Geometry check sheet. Reference: the model listing, model coordinates, mm. Coordinates: 2 decimals unless noted, no trailing zeros. Write each loop counter-clockwise with the first axis right and the second up, starting at its lowest first coordinate (ties: lowest second). Pieces come first, ordered by that corner, then holes. Notation, with made-up numbers: (-25.5, -27.5) -> (-15.5, -27.5) arc R22 cw to (-15.5, -13.5) -> close; hole circle Ø11 at (70, 55). An arc over 180 degrees is marked (long way). One line per question, with ' | ' between items.
from build123d import *

# Parameters (mm, degrees)
SKETCH1_W           = 145
SKETCH1_H           = 155
BOSS_EXTRUDE1_DEPTH = 3
SKETCH3_W           = 4.5
SKETCH3_H           = 4
CUT_EXTRUDE1_DEPTH  = 3
SKETCH4_R           = 2.05
CUT_EXTRUDE2_DEPTH  = 3
SKETCH5_R           = 2.05
CUT_EXTRUDE3_DEPTH  = 10


with BuildPart() as part:
    # Sketch1 → Boss-Extrude1 (new body)
    with BuildSketch(Plane(origin=(0, 0, 0), x_dir=(1, 0, 0), z_dir=(0, 1, 0))):
        Rectangle(SKETCH1_W, SKETCH1_H)
    extrude(amount=BOSS_EXTRUDE1_DEPTH)

    # Sketch3 → Cut-Extrude1 (cut)
    with BuildSketch(Plane(origin=(0, 3, 0), x_dir=(1, 0, 0), z_dir=(0, 1, 0))):
        Polygon((-61.5, -37), (-72.5, -37), (-72.5, -77.5), (-61.5, -77.5), (-61.5, -73.5), align=None)
        with Locations((-59.25, -75.5)):
            Rectangle(SKETCH3_W, SKETCH3_H)
    extrude(amount=-CUT_EXTRUDE1_DEPTH, mode=Mode.SUBTRACT)

    # Sketch4 → Cut-Extrude2 (cut)
    with BuildSketch(Plane(origin=(0, 3, 0), x_dir=(1, 0, 0), z_dir=(0, 1, 0))):
        with Locations(Location((-17.5, -67.5, 0), (0, 0, 270))):
            Circle(SKETCH4_R)
        with Locations(Location((62.5, -67.5, 0), (0, 0, 270))):
            Circle(SKETCH4_R)
        with Locations(Location((-62.5, -22.85, 0), (0, 0, 270))):
            Circle(SKETCH4_R)
        with Locations(Location((-62.5, 57.15, 0), (0, 0, 270))):
            Circle(SKETCH4_R)
        with Locations(Location((62.5, -47.5, 0), (0, 0, 270))):
            Circle(SKETCH4_R)
        with Locations(Location((-17.5, -47.5, 0), (0, 0, 270))):
            Circle(SKETCH4_R)
    extrude(amount=-CUT_EXTRUDE2_DEPTH, mode=Mode.SUBTRACT)

    # Sketch5 → Cut-Extrude3 (cut)
    with BuildSketch(Plane(origin=(0, 3, 0), x_dir=(1, 0, 0), z_dir=(0, 1, 0))):
        with Locations(Location((52.538287268, 25.128851924, 0), (0, 0, 270))):
            Circle(SKETCH5_R)
        with Locations(Location((-14.95509898, 16.575946892, 0), (0, 0, 270))):
            Circle(SKETCH5_R)
    extrude(amount=-CUT_EXTRUDE3_DEPTH, mode=Mode.SUBTRACT)


solid = part.part
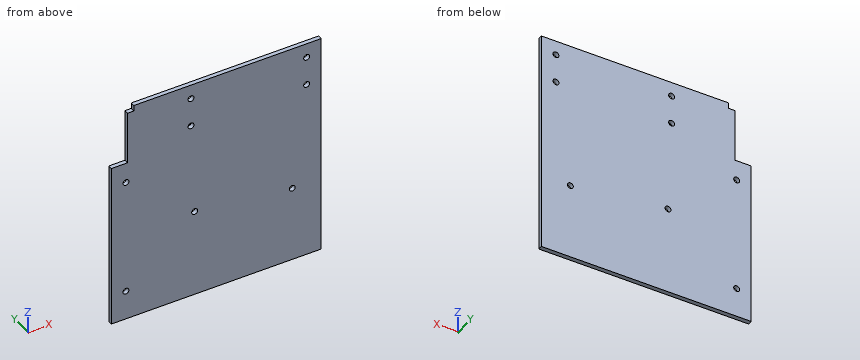
1. Cross-section at B-B on z = 47.5. Record the boundary of the cut face in (x, y).
Worked answers:
outline: (-61.5, 0) -> (-19.55, 0) -> (-19.55, 3) -> (-61.5, 3) -> close; (-15.45, 0) -> (60.45, 0) -> (60.45, 3) -> (-15.45, 3) -> close; (64.55, 0) -> (72.5, 0) -> (72.5, 3) -> (64.55, 3) -> close
2. Cross-section at A-A on x = 62.5. Record the boundary of the cut face in (y, z).
Worked answers:
outline: (0, -77.5) -> (3, -77.5) -> (3, 45.45) -> (0, 45.45) -> close; (0, 49.55) -> (3, 49.55) -> (3, 65.45) -> (0, 65.45) -> close; (0, 69.55) -> (3, 69.55) -> (3, 77.5) -> (0, 77.5) -> close
3. Material ranges on line 1 (X direction, y = 2.3, z = 47.5); line 2 (X direction, y = 2.15, z = 22.85); line 3 (Z direction, x = -64, y = 2.5), recorded low to high. Write a range as from..to.
Worked answers:
line 1: -61.5..-19.55, -15.45..60.45, 64.55..72.5 | line 2: -72.5..-64.55, -60.45..72.5 | line 3: -77.5..-58.55, -55.75..21.45, 24.25..37
4. Cross-section at C-C on z = 22.85. Record the boundary of the cut face in (x, y), and give its area (3 significant figures).
Worked answers:
outline: (-72.5, 0) -> (-64.55, 0) -> (-64.55, 3) -> (-72.5, 3) -> close; (-60.45, 0) -> (72.5, 0) -> (72.5, 3) -> (-60.45, 3) -> close | area: 423 mm²
5. Go/stop test with flat-tipped pins: P1, Ø1.5, axis at y = 2, z = 76.5, coming from the -X side; P2, Ø1.5, axis at x = -59, y = 1, coming from the +Z side. Record where each tip stops, or that it passes through.
Worked answers:
P1: x = -57 | P2: z = 73.5
6. Cross-section at D-D on y = 2.05. Give the number of separate pieces and of enclosed holes in the cut face, and give its area (3 significant figures).
Worked answers:
separate pieces: 1 | enclosed holes: 8 | area: 21,900 mm²
